Read the model definition and answer for the solid it produces. Units are mm, in the model's axes. Face numbers are marked on the shaded views. A direction names the side the tool comes from. Coordinates: 2 decimals unless noted, no trailing zeros. Write each loop counter-clockwise with the first axis right and the second up, starting at its lowest first coordinate (ties: lowest second). Pieces come first, ordered by that corner, then holes. Notation, with made-up numbers: M 38.5,34.5 L 68.5,34.5 A7 cw 68.5,41.5 Z; hole C -4,27 d1. An arc over 180 degrees is marked long. Use a Markdown table: item, result. Add a question column.
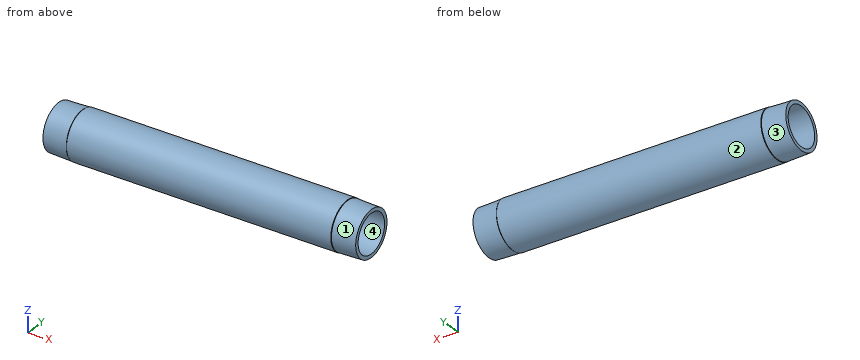
Autodesk Inventor part; units mm, degrees
ref_plane "YZ Plane" through (0, 0, 0) normal (1, 0, 0) x (0, 1, 0)
ref_plane "XZ Plane" through (0, 0, 0) normal (0, 1, 0) x (-1, 0, 0)
ref_plane "XY Plane" through (0, 0, 0) normal (0, 0, 1) x (1, 0, 0)
sketch "スケッチ1" plane through (0, 0, 0) normal (0, 0, 1) x (1, 0, 0)
  line L0 (-110.39, 0) -> (110.39, 0)
  line L1 (-110.39, 0) -> (-110.39, 17)
  line L2 (-110.39, 17) -> (110.39, 17)
  line L3 (110.39, 0) -> (110.39, 17)
  line L4 (-110.39, 13.8) -> (110.39, 13.8)
  point P0 (0, 0)
  point P1 (0, 0)
  dimension "d0" = 34
  dimension "d1" = 3.2
  dimension "d2" = 220.78
revolve "回転1" add sketch "スケッチ1" angle 360 about axis through (-110.39, 0, 0) along (1, 0, 0) contours L1 L2 L3 L4
sketch "スケッチ2" plane through (0, 0, 0) normal (0, 0, 1) x (1, 0, 0)
  line L0 (-110.39, 17) -> (110.39, 17)
  line L1 (-110.39, -17) -> (-110.39, 17)
  line L2 (-110.39, 16.2998) -> (-93.6, 16.8245)
  line L3 (-93.6, 16.8245) -> (-93.296, 17)
  line L4 (-110.39, 0) -> (57.6085, 0)
  line L5 (-100, 16.6245) -> (-100, 0) construction
  point P0 (0, 0)
  dimension "d4" = 33.249
  dimension "d5" = 1.79
  dimension "d6" = 10.39
  dimension "d9" = 30
  dimension "d10" = 6.4
revolve "回転2" cut sketch "スケッチ2" angle 360 about axis through (-110.39, 0, 0) along (1, 0, 0)
thread "ねじ1【手修正】"
mirror "ミラー1" about plane through (0, 0, 0) normal (1, 0, 0) of "回転2"
thread "ねじ2【手修正】"
ref_plane "作業平面1" through (-100, 0, 0) normal (-1, 0, 0) x (0, 0, 1)
ref_plane "作業平面2" through (100, 0, 0) normal (1, 0, 0) x (0, 0, -1)
equation "\"d0\" = DIA"
equation "\"d1\" = T1"
equation "\"d2\" = length + 2 * L1"
equation "\"d4\" = DIA_1"
equation "\"d6\" = L1"
equation "\"d10\" = L2"
equation "\"DIA\" = 34"
equation "\"T1\" = 3.2"
equation "\"DIA_1\" = 33.249"
equation "\"L1\" = 10.39"
equation "\"L2\" = 6.4"
equation "\"length\" = 200"
equation "\"d16\" = -L1"
equation "\"d17\" = -L1"
properties part number "Threaded pipe_SGP._1ipt" material "SS400"
Item 1: Find section C-C on x = -47. Give the vertices of the cut face in (y, z), then the cut area to 3 significant figures.
Item 2: Each of these flat-tipped pins is pushed along its axis until it touches: pin 1 (5 mm diameter, centred on x = -5, z = -6.5, fed in from +Y); pin 2 (2 mm diameter, centred on x = -77, y = 8.5, fed in from -Z); pin 3 (3 mm diameter, centred on x = -3.5, y = -11, fed in from -Z). Where does it stop, or does it pass through?
Item 3: For the marked faces 1 and 2, determine the directions among +Z, -Z, +X, -X, +Y, -Y from which every point of the face is accessible in a straight line to the end or side of a thin tool.
Item 4: Consider probe 1 along Y at (x, z) = (-6, -0.5); probe 2 along Z at (x, y) = (-6, 0); probe 3 along Y at (x, z) = (92, 10). Determine where each line is inside the solid, lowest interval first.
Item 5: Determine the mould class of the marked faces 3 and 4 for opening direction Y: pulls with the +Y half, pulls with the -Y half, needs draft (parallel to the pull), parting line crosses it, or undercut.
Item 6: Find section A-A on y = 0. Give the vertices of the cut face in (x, z), then the cut area to 3 significant figures.
Geometry says:
| question | item | result |
|---|---|---|
| 1 | outline | C 0,0 d34; hole C 0,0 d27.6 |
| 1 | area | 310 mm2 |
| 2 | pin 1 | stops at y = 16.52 |
| 2 | pin 2 | stops at z = -15.26 |
| 2 | pin 3 | stops at z = -14.1 |
| 3 | face 1 | +X |
| 3 | face 2 | +X, -X |
| 4 | probe 1 | y = -16.99 to -13.79, 13.79 to 16.99 |
| 4 | probe 2 | z = -17 to -13.8, 13.8 to 17 |
| 4 | probe 3 | y = -13.75 to -9.51, 9.51 to 13.75 |
| 5 | face 3 | parting line crosses it |
| 5 | face 4 | undercut |
| 6 | outline | M -110.39,-16.3 L -93.6,-16.82 L -93.3,-17 L 93.3,-17 L 93.6,-16.82 L 110.39,-16.3 L 110.39,-13.8 L -110.39,-13.8 Z; M -110.39,13.8 L 110.39,13.8 L 110.39,16.3 L 93.6,16.82 L 93.3,17 L -93.3,17 L -93.6,16.82 L -110.39,16.3 Z |
| 6 | area | 1,380 mm2 |
